The listing builds one solid part. Answer for the finished solid, in the listing's coordinates (mm). Face numbers are marked on the shaded views. A direction names the side the tool comes from. Give positions to 0.01 mm unless a question says otherwise; leave off trailing zeros. Order: outer loops, then holes, each group sorted by start corner. A loop starts at its lowest first (then second) coordinate and runs counter-clockwise, first axis right, second up. Notation, with made-up numbers: (-21.75, 7) - (-4.75, 7) arc R27 cw to (-4.75, 36) - close; hole circle Ø6 at (14, 70). An arc over 180 degrees is marked (long way). Use CSV: the item, a comma, the result in double quotes.
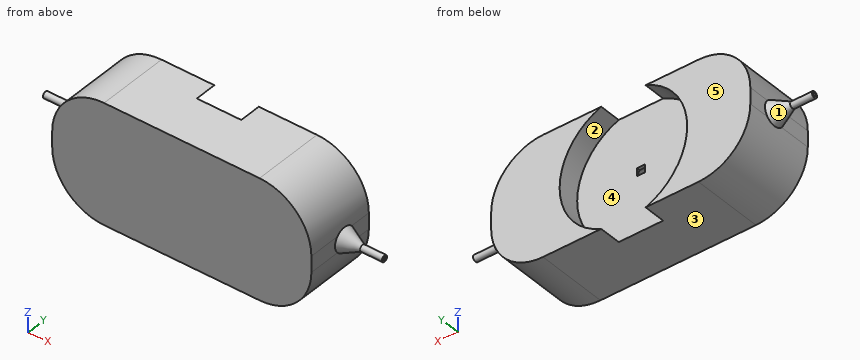
```python
from build123d import *

# Parameters (mm, degrees)
SKETCH1_W           = 65
SKETCH1_H           = 30
BOSS_EXTRUDE1_DEPTH = 58
FILLET1_R           = 13
SKETCH15_W          = 83.696095513
SKETCH15_H          = 31.69844841
CUT_EXTRUDE7_DEPTH  = 50
SKETCH18_R          = 16
CUT_EXTRUDE10_DEPTH = 5.5
CUT_EXTRUDE12_REACH = 90.397
SKETCH3_R           = 1.6
SKETCH21_W          = 2
SKETCH21_H          = 2
CUT_EXTRUDE13_DEPTH = 8


with BuildPart() as part:
    # Sketch1 → Boss-Extrude1 (new body)
    with BuildSketch(Plane(origin=(0, 0, 0), x_dir=(1, 0, 0), z_dir=(0, 1, 0))):
        with Locations((7.5, 0)):
            Rectangle(SKETCH1_W, SKETCH1_H)
    extrude(amount=BOSS_EXTRUDE1_DEPTH)

    # Fillet1
    fillet1_edges = [part.edges().sort_by_distance(p)[0] for p in [
        (40, 29, 15),
        (-25, 29, 15),
        (-25, 29, -15),
        (40, 29, -15),
    ]]
    fillet(fillet1_edges, radius=FILLET1_R)

    # Sketch15 → Cut-Extrude7 (cut)
    with BuildSketch(Plane(origin=(0, -10, 0), x_dir=(-1, 0, 0), z_dir=(0, -1, 0))):
        with Locations((-0.057440767, 0.030479277)):
            Rectangle(SKETCH15_W, SKETCH15_H)
    extrude(amount=-CUT_EXTRUDE7_DEPTH, mode=Mode.SUBTRACT)

    # Sketch18 → Cut-Extrude10 (cut)
    with BuildSketch(Plane(origin=(0, 58, 0), x_dir=(1, 0, 0), z_dir=(0, 1, 0))):
        with Locations((6.828508286, 0)):
            Circle(SKETCH18_R)
    extrude(amount=-CUT_EXTRUDE10_DEPTH, mode=Mode.SUBTRACT)

    # Sketch3 → Cut-Extrude12 (cut, up to next)
    with BuildSketch(Plane.ZY.offset(25), mode=Mode.PRIVATE) as cut_extrude12_sk1:
        with Locations((0, 50.4)):
            Circle(SKETCH3_R)
    cut_extrude12_tool1 = extrude(cut_extrude12_sk1.sketch, amount=-CUT_EXTRUDE12_REACH, mode=Mode.PRIVATE) & part.part
    add(cut_extrude12_tool1.solids().sort_by_distance((-25, 50.4, 0))[0], mode=Mode.SUBTRACT)

    # Sketch21 → Cut-Extrude13 (cut)
    with BuildSketch(Plane(origin=(0, 52.5, 0), x_dir=(1, 0, 0), z_dir=(0, 1, 0))):
        with Locations((6.828508286, 0)):
            Rectangle(SKETCH21_W, SKETCH21_H)
    extrude(amount=-CUT_EXTRUDE13_DEPTH, mode=Mode.SUBTRACT)

    # Sketch24 → Revolve1 (revolve)
    with BuildSketch(Plane.XY, mode=Mode.PRIVATE) as revolve1_sk:
        Polygon((-25, 50.8), (-35, 50.8), (-35, 51.2), (-29.5, 51.2), (-25, 53.4), align=None)
    revolve(revolve1_sk.sketch.rotate(Axis((-25, 50.4, 0), (-1, 0, 0)), 90), axis=Axis((-25, 50.4, 0), (-1, 0, 0)))

    # Sketch25 → Revolve2 (revolve)
    with BuildSketch(Plane.XY, mode=Mode.PRIVATE) as revolve2_sk:
        Polygon((40, 50.79856611), (40, 53.39856611), (44.5, 51.19856611), (50, 51.19856611), (50, 50.79856611), align=None)
    revolve(revolve2_sk.sketch.rotate(Axis((50.482197819, 50.39856611, 0), (-1, 0, 0)), 90), axis=Axis((50.482197819, 50.39856611, 0), (-1, 0, 0)))


solid = part.part
```
Item 1: Which of the six approach directions +Z, -Z, +X, -X, +Y, -Y give full straight-line access (tool end or side, diameter ignored) to the marked faces 1 and 2?
Taken from the geometry:
face 1,"-X"
face 2,"+Y"
Item 2: The mould has two halves that part along Z. Classify the marked faces 3, 4 and 5: +Z half, -Z half, draft (parallel to the pull), parting line (faces both ways), or undercut.
Taken from the geometry:
face 3,"-Z half"
face 4,"undercut"
face 5,"draft"
Item 3: The part is cut by section D-D (z = 5.5). Give the vertices of the cut face in (x, y).
Taken from the geometry:
outline,"(-24.52, 40) - (39.52, 40) - (39.52, 58) - (21.85, 58) - (21.85, 52.5) - (-8.2, 52.5) - (-8.2, 58) - (-24.52, 58) - close"
Item 4: The part is cut by section C-C (x = -20). Give the vertices of the cut face in (y, z).
Taken from the geometry:
outline,"(40, -12.25) - (58, -12.25) - (58, 12.25) - (40, 12.25) - close; hole circle Ø3.2 at (50.4, 0)"
Item 5: Each of these flat-tipped pins is pushed along its axis until it touches: pin 1 (8 mm diameter, centred on y = 55, z = 6.5, fed in from +X); pin 2 (2 mm diameter, centred on y = 46, z = -0.5, fed in from -X); pin 3 (0.8 mm diameter, centred on y = 51.5, z = 2.5, fed in from -X). Where does it stop, or does it pass through?
Taken from the geometry:
pin 1,"x = 39.99"
pin 2,"x = -25"
pin 3,"x = -26.37"
Item 6: The part is cut by section B-B (y = 46.25). Give the vertices of the cut face in (x, z), and give its area (3 significant figures).
Taken from the geometry:
outline,"(-25, -2) arc R13 ccw to (-12, -15) - (27, -15) arc R13 ccw to (40, -2) - (40, 2) arc R13 ccw to (27, 15) - (-12, 15) arc R13 ccw to (-25, 2) - close; hole (5.83, -1) - (7.83, -1) - (7.83, 1) - (5.83, 1) - close"
area,"1,800 mm^2"
Item 7: Find the intervals of material crossed by line 1 along X through (y, z) = (45, 0); line 2 along Y through (x, z) = (-1, 0); line 3 along X through (y, z) = (50, -0.5), in increasing order.
Taken from the geometry:
line 1,"-25 to 5.83, 7.83 to 40"
line 2,"40 to 48.8, 52 to 52.5"
line 3,"-35 to -25, 40 to 50"
Item 8: The part is cut by section A-A (y = 42.75). Give the vertices of the cut face in (x, z).
Taken from the geometry:
outline,"(-25, -2) arc R13 ccw to (-12, -15) - (27, -15) arc R13 ccw to (40, -2) - (40, 2) arc R13 ccw to (27, 15) - (-12, 15) arc R13 ccw to (-25, 2) - close"
